Model file for the job. Use its own axes, mm. A direction names the side the tool comes from. Round coordinates to 2 decimals unless told otherwise and drop trailing zeros. Order: outer loops, then holes, each group sorted by start corner. A loop starts at its lowest first (then second) coordinate and runs counter-clockwise, first axis right, second up. Notation, with made-up numbers: M 68,5.5 L 82,5.5 A8 cw 82,17.5 Z; hole C 57.5,-19.5 d6. An arc over 180 degrees is marked long. Return JSON: item names as keys, results as strings. Group by question number.
Item 1: Which spindle directions (+Z, -Z, +X, -X, +Y, -Y) get a long thin tool onto all of the face, cutting with end or side? Do faces 4 (the face through (-11, -18, 0)), 5 (the face through (-8.5, -10, 0)), 6 (the face through (-14.25, -5, 0)). Say none if no direction does.
Item 2: Probe line 1 along X through (y, z) = (-17.35, -0.6) (3 decimals); line 2 along Y through (x, z) = (-7.5, 0.3); line 3 along X through (y, z) = (-2, -0.35). List the from-to ranges inside material, lowest first.
Item 3: Slice it at D-D on y = -17.35. Write the cut outline in (x, z) (3 decimals).
Item 4: Pull direction X, two halves, no side cores. Call faces 1 (the face through (14.25, -5, 0)), 2 (the face through (0, 0, 0)), 3 (the face through (0, 2, -0.781)): pulls with the +X half, pulls with the -X half, needs draft (parallel to the pull), parting line crosses it, or undercut.
Item 5: Slice it at B-B on x = 7.5. Write the cut outline in (y, z), then the cut area to 3 significant figures.
Item 6: Pin check, flat tips, straight feed: pin 1 Ø0.6 at (x, z) = (-11, 0.5) entering from -Y; pin 2 Ø3 at (x, y) = (12, -18) entering from +Z. Stop position of each tip, or through.
Item 7: Slice it at C-C on z = 0.25. Write the cut outline in (x, y).
Item 8: Slice it at A-A on y = -12.75. Write the cut outline in (x, z).
from build123d import *

# Parameters (mm, degrees)
SKETCH1_R           = 1
SKETCH1_R_2         = 0.5
BOSS_EXTRUDE1_DEPTH = 0.781250025
SKETCH2_W           = 5.75
SKETCH2_H           = 4
CUT_EXTRUDE1_DEPTH  = 0.781250025


with BuildPart() as part:
    # Sketch1 → Boss-Extrude1 (new, symmetric)
    with BuildSketch(Plane.XY):
        Polygon((-8.5, -19.85), (-8.5, 0), (8.5, 0), (8.5, -19.85), (14.25, -19.85), (14.25, 10), (-14.25, 10), (-14.25, -19.85), align=None)
        with Locations((-7.5, 5)):
            Circle(SKETCH1_R, mode=Mode.SUBTRACT)
        with Locations((7.5, 5)):
            Circle(SKETCH1_R, mode=Mode.SUBTRACT)
        with Locations((-11.375, -17.35)):
            Circle(SKETCH1_R_2, mode=Mode.SUBTRACT)
        with Locations((11.375, -17.35)):
            Circle(SKETCH1_R_2, mode=Mode.SUBTRACT)
    extrude(amount=BOSS_EXTRUDE1_DEPTH, both=True)

    # Sketch2 → Cut-Extrude1 (cut)
    with BuildSketch(Plane.XY.offset(0.781250025)):
        with Locations((-11.375, -17.85)):
            Rectangle(SKETCH2_W, SKETCH2_H)
        with Locations((11.375, -17.85)):
            Rectangle(SKETCH2_W, SKETCH2_H)
    extrude(amount=-CUT_EXTRUDE1_DEPTH, mode=Mode.SUBTRACT)


solid = part.part
Output values:
{
 "1": {"face 4": "+Z, +X, -X, -Y", "face 5": "+Z, -Z, -Y", "face 6": "+Z, -Z, -X, +Y, -Y"},
 "2": {"line 1": "-14.25 to -11.875, -10.875 to -8.5, 8.5 to 10.875, 11.875 to 14.25", "line 2": "0 to 4, 6 to 10", "line 3": "-14.25 to -8.5, 8.5 to 14.25"},
 "3": {"outline": "M -14.25,-0.781 L -11.875,-0.781 L -11.875,0 L -14.25,0 Z; M -10.875,-0.781 L -8.5,-0.781 L -8.5,0 L -10.875,0 Z; M 8.5,-0.781 L 10.875,-0.781 L 10.875,0 L 8.5,0 Z; M 11.875,-0.781 L 14.25,-0.781 L 14.25,0 L 11.875,0 Z"},
 "4": {"face 1": "pulls with the +X half", "face 2": "undercut", "face 3": "needs draft"},
 "5": {"outline": "M 0,-0.78 L 4,-0.78 L 4,0.78 L 0,0.78 Z; M 6,-0.78 L 10,-0.78 L 10,0.78 L 6,0.78 Z", "area": "12.5 mm²"},
 "6": {"pin 1": "y = -15.85", "pin 2": "z = 0"},
 "7": {"outline": "M -14.25,-15.85 L -8.5,-15.85 L -8.5,0 L 8.5,0 L 8.5,-15.85 L 14.25,-15.85 L 14.25,10 L -14.25,10 Z; hole C -7.5,5 d2; hole C 7.5,5 d2"},
 "8": {"outline": "M -14.25,-0.78 L -8.5,-0.78 L -8.5,0.78 L -14.25,0.78 Z; M 8.5,-0.78 L 14.25,-0.78 L 14.25,0.78 L 8.5,0.78 Z"}
}
